Part model, mm, in its own coordinate system. A direction names the side the tool comes from. Give positions to 0.01 mm unless a question says otherwise; leave off trailing zeros. Order: outer loops, then holes, each group sorted by start corner. A loop starts at its lowest first (then second) coordinate and runs counter-clockwise, first axis right, second up. Notation, with made-up numbers: M 85.5,58 L 140.5,58 A14 cw 140.5,79 Z; hole C 53,84.5 d7. An arc over 180 degrees is marked long. Return JSON: item names as keys, results as strings.
from build123d import *

# Parameters (mm, degrees)
SKETCH001_W     = 15
SKETCH001_H     = 7
PAD_DEPTH       = 9
SKETCH_R        = 2.55
POCKET_DEPTH    = 7
SKETCH002_R     = 0.6
POCKET001_DEPTH = 5


with BuildPart() as part:
    # Sketch001 → Pad (new body)
    with BuildSketch(Plane(origin=(0, 0, 0), x_dir=(1, 0, 0), z_dir=(0, 0, -1))):
        with Locations((0.536015, 2.732478)):
            Rectangle(SKETCH001_W, SKETCH001_H)
    extrude(amount=PAD_DEPTH)

    # Sketch → Pocket (cut)
    with BuildSketch(Plane(origin=(0, 0, -9), x_dir=(1, 0, 0), z_dir=(0, 0, -1))):
        with Locations((-3.254865, 2.67761)):
            Circle(SKETCH_R)
        with Locations((4.144291, 2.789385)):
            Circle(SKETCH_R)
    extrude(amount=-POCKET_DEPTH, mode=Mode.SUBTRACT)

    # Sketch002 → Pocket001 (cut)
    with BuildSketch(Plane(origin=(0, 0, -2), x_dir=(1, 0, 0), z_dir=(0, 0, -1))):
        with Locations((-3.213175, 2.787703)):
            Circle(SKETCH002_R)
        with Locations((4.18651, 2.825651)):
            Circle(SKETCH002_R)
    extrude(amount=-POCKET001_DEPTH, mode=Mode.SUBTRACT)


solid = part.part
Q1. 3-axis set-ups, long thin cutter, end or side, ignore diameter. For faces 4 (the cylindrical face through (-3.813, -2.814, -1.014)), 5 (the cylindrical face through (-2.078, -0.415, -5.549)): which of +Z, -Z, +X, -X, +Y, -Y reach the whole face in a straight line?
Established:
{"face 4": "+Z, -Z", "face 5": "-Z"}
Q2. Band-saw the part on B-B (x = -3). Give the cut face in (y, z), then the cut area to 3 significant figures.
Established:
{"outline": "M -6.23,-9 L -5.21,-9 L -5.21,-2 L -3.35,-2 L -3.35,0 L -6.23,0 Z; M -2.23,-2 L -0.14,-2 L -0.14,-9 L 0.77,-9 L 0.77,0 L -2.23,0 Z", "area": "25.2 mm²"}
Q3. Probe line 1 along X through (y, z) = (-3, -1.5); line 2 along X through (y, z) = (-0.5, -2.75); line 3 along Z through (x, y) = (3, -2). List the from-to ranges inside material, lowest first.
Established:
{"line 1": "x = -6.96 to -3.77, -2.65 to 3.61, 4.76 to 8.04", "line 2": "x = -6.96 to -4.58, -1.93 to 3.02, 5.27 to 8.04", "line 3": "z = -2 to 0"}
Q4. Pin check, flat tip, straight feed: pin 1 (1.5 mm diameter, centred on x = 3, y = -2, fed in from -Z). Stop position of the tip, or through.
Established:
{"pin 1": "stops at z = -2"}
Q5. Band-saw the part on D-D (y = -4). Give the cut face in (x, z), then the cut area to 3 significant figures.
Established:
{"outline": "M -6.96,-9 L -5.44,-9 L -5.44,-2 L -1.07,-2 L -1.07,-9 L 1.9,-9 L 1.9,-2 L 6.39,-2 L 6.39,-9 L 8.04,-9 L 8.04,0 L -6.96,0 Z", "area": "73.1 mm²"}
Q6. Two-plate mould, pull along X, no slides. Class faces 1 (the flat face through (0, -3, -9)), 2 (the flat face through (8.036, -3, -4)), 3 (the cylindrical face through (3.587, -2.852, -1.014)): +X half, -X half, draft (parallel to the pull), parting line (faces both ways), or undercut.
Established:
{"face 1": "draft", "face 2": "+X half", "face 3": "undercut"}
Q7. Band-saw the part on C-C (z = -5.5). Give the cut face in (x, y), then the cut area to 3 significant figures.
Established:
{"outline": "M -6.96,-6.23 L 8.04,-6.23 L 8.04,0.77 L -6.96,0.77 Z; hole C -3.25,-2.68 d5.1; hole C 4.14,-2.79 d5.1", "area": "64.1 mm²"}
Q8. Band-saw the part on A-A (y = -3). Give the cut face in (x, z), then the cut area to 3 significant figures.
Established:
{"outline": "M -6.96,-9 L -5.78,-9 L -5.78,-2 L -3.77,-2 L -3.77,0 L -6.96,0 Z; M -2.65,-2 L -0.73,-2 L -0.73,-9 L 1.6,-9 L 1.6,-2 L 3.61,-2 L 3.61,0 L -2.65,0 Z; M 4.76,-2 L 6.69,-2 L 6.69,-9 L 8.04,-9 L 8.04,0 L 4.76,0 Z", "area": "59.5 mm²"}
